from build123d import *

# Parameters (mm, degrees)
F0_W     = 798.5125
F0_H     = 1295.4
F1_DEPTH = 355.6
F2_DEPTH = 328.5871
F3_SIZE  = 6.35
F4_SIZE  = 6.35


with BuildPart() as f1:
    # F0 (on Front) → F1 (new body)
    with BuildSketch(Plane.XZ):
        Rectangle(F0_W, F0_H)
        Polygon((323.05625, 571.5), (323.05625, 323.85), (323.05625, -69.85), (-323.05625, -69.85), (-323.05625, 571.5), align=None, mode=Mode.SUBTRACT)
    extrude(amount=F1_DEPTH)

    # F0 (on Front) → F2 (join)
    with BuildSketch(Plane.XZ):
        Polygon((323.05625, -69.85), (323.05625, 323.85), (323.05625, 571.5), (-323.05625, 571.5), (-323.05625, -69.85), align=None)
    extrude(amount=F2_DEPTH)

    # F3
    f3_edges = [f1.edges().sort_by_distance(p)[0] for p in [
        (0, -355.6, -69.85),
        (-323.05625, -355.6, 250.825),
        (0, -355.6, 571.5),
        (323.05625, -355.6, 250.825),
    ]]
    chamfer(f3_edges, length=F3_SIZE)

    # F4
    f4_edges = [f1.edges().sort_by_distance(p)[0] for p in [
        (399.25625, -355.6, 0),
        (0, -355.6, 647.7),
        (-399.25625, -355.6, 0),
        (-399.25625, -177.8, 647.7),
        (399.25625, -177.8, 647.7),
        (-399.25625, 0, 0),
        (399.25625, 0, 0),
    ]]
    chamfer(f4_edges, length=F4_SIZE)


solid = f1.part
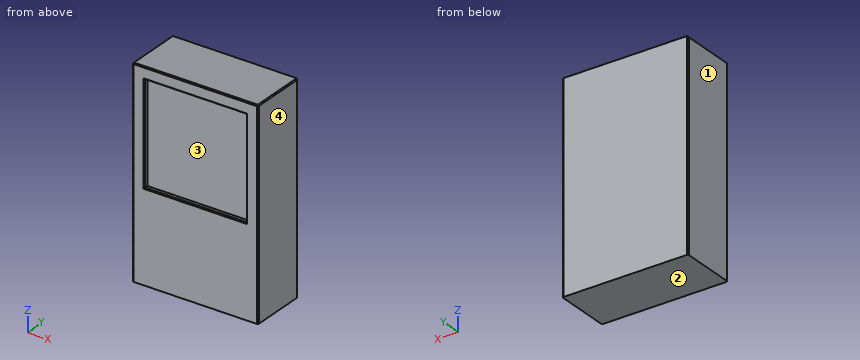
Input: part model. Units: mm. Frame: model coordinates. Face numbers are marked on the shaded views. Coordinates: 2 decimals unless noted, no trailing zeros. Loops run counter-clockwise (first coordinate to the right, second up) from the corner with the lowest first, then second, coordinate; pieces in that order, holes last.
Q1. Material intervals for line 1 (Z direction, x = -241.5, y = -335.5); line 2 (Y direction, x = -98.5, z = 155.5), sorted ascending.
Q2. Draft query along X for the marked faces 1, 2, 3 and 4. Return one class per face: +X half, -X half, draft (parallel to the pull), parting line (faces both ways), or undercut.
Q3. Cut plane A-A (z = 212.5). Output: boundary loops of the cut face in (x, y), then the cut area to 3 significant figures.
Q4. Cut plane B-B (x = -36.5). Output: boundary loops of the cut face in (y, z), then the cut area to 3 significant figures.
Working result:
1. line 1: z = -647.7 to -69.85, 571.5 to 647.7
1. line 2: y = -328.59 to 0
2. face 1: -X half
2. face 2: draft
2. face 3: undercut
2. face 4: +X half
3. outline: (-399.26, -349.25) - (-392.91, -355.6) - (-329.41, -355.6) - (-323.06, -349.25) - (-323.06, -328.59) - (323.06, -328.59) - (323.06, -349.25) - (329.41, -355.6) - (392.91, -355.6) - (399.26, -349.25) - (399.26, -6.35) - (392.91, 0) - (-392.91, 0) - (-399.26, -6.35) - close
3. area: 266,000 mm2
4. outline: (-355.6, -647.7) - (0, -647.7) - (0, 647.7) - (-349.25, 647.7) - (-355.6, 641.35) - (-355.6, 577.85) - (-349.25, 571.5) - (-328.59, 571.5) - (-328.59, -69.85) - (-349.25, -69.85) - (-355.6, -76.2) - close
4. area: 443,000 mm2
